```python
from build123d import *

# Parameters (mm, degrees)
SKETCH_2_R   = 5
SKETCH_2_R_2 = 2.092708753


with BuildPart() as part:
    # 扫描1: sweep along a path in 草图1
    with BuildLine(Plane.XY) as sweep_1_path:
        Line((0, 0), (0, 12))
        ThreePointArc((0, 12), (2.343145751, 17.656854249), (8, 20))
        Line((8, 20), (20, 20))
    # 草图2 → 扫描1 (sweep)
    with BuildSketch(Plane(origin=(0, 0, 0), x_dir=(1, 0, 0), z_dir=(0, 1, 0))):
        Circle(SKETCH_2_R)
        Circle(SKETCH_2_R_2, mode=Mode.SUBTRACT)
    sweep(path=sweep_1_path.line)


solid = part.part
```
Geometry: final body of the model. Coordinates: model frame, mm. A direction names the side the tool comes from. Coordinates: 2 decimals unless noted, no trailing zeros. Order: outer loops, then holes, each group sorted by start corner. A loop starts at its lowest first (then second) coordinate and runs counter-clockwise, first axis right, second up. Notation, with made-up numbers: (-34, -34.5) -> (6, -34.5) arc R20 ccw to (6, -27.5) -> close; hole circle Ø1 at (86.5, 54.5). An arc over 180 degrees is marked (long way). Answer in a Markdown table with one row per item.
Item 1: Section C-C on z = 3.5. Output: boundary loops of the cut face in (x, y).
Return value:
| item | result |
|---|---|
| outline | (-3.57, 0) -> (3.57, 0) -> (3.57, 12) arc R4.43 cw to (8, 16.43) -> (20, 16.43) -> (20, 23.57) -> (8, 23.57) arc R11.57 ccw to (-3.57, 12) -> close |
Item 2: Access query for faces 1 (the cylindrical face through (14, 25, 0)), 2 (the cylindrical face through (-0.454, 6.084, 2.043)). Directions: +Z, -Z, +X, -X, +Y, -Y. A direction counts if a zero-diameter tool reaches every point of the face in a straight line with its end or side. Return the directions, or none.
Return value:
| item | result |
|---|---|
| face 1 | +X |
| face 2 | -Y |
Item 3: Contact query for flat-ended pins moving along their axis: P1, Ø6, axis at y = 21.5, z = 0.5, coming from the -X side; P2, Ø4, axis at x = 0, z = 0, coming from the +Y side; P3, Ø1, axis at y = 19.5, z = 0, coming from the +X side; P4, Ø6, axis at y = 2.5, z = 2.5, coming from the -X side. Output: stop coordinate, or through.
Return value:
| item | result |
|---|---|
| P1 | stops at x = -3.25 |
| P2 | stops at y = 23.53 |
| P3 | stops at x = 1.85 |
| P4 | stops at x = -5 |
Item 4: Draft query along Y for faces 3 (the flat face through (-2.2, 0, 1)), 4 (the flat face through (20, 22.2, 1)), 5 (the cylindrical face through (14.08, 22.09, -0.09)). Return one class per face: released by +Y, released by -Y, zero draft, split by the parting line, or undercut.
Return value:
| item | result |
|---|---|
| face 3 | released by -Y |
| face 4 | zero draft |
| face 5 | undercut |
Item 5: Section A-A on z = 0. Output: boundary loops of the cut face in (x, y).
Return value:
| item | result |
|---|---|
| outline | (-5, 0) -> (-2.09, 0) -> (-2.09, 12) arc R10.09 cw to (8, 22.09) -> (20, 22.09) -> (20, 25) -> (8, 25) arc R13 ccw to (-5, 12) -> close; (2.09, 0) -> (5, 0) -> (5, 12) arc R3 cw to (8, 15) -> (20, 15) -> (20, 17.91) -> (8, 17.91) arc R5.91 ccw to (2.09, 12) -> close |
Item 6: Ray query, L1, parallel to X at y = 3, z = 0; L2, parallel to Y at x = 11, z = 0. Return the intervals inside material, ascending.
Return value:
| item | result |
|---|---|
| L1 | x = -5 to -2.09, 2.09 to 5 |
| L2 | y = 15 to 17.91, 22.09 to 25 |
Item 7: Section B-B on x = 8.5. Output: boundary loops of the cut face in (y, z).
Return value:
| item | result |
|---|---|
| outline | circle Ø10 at (20, 0); hole circle Ø4.19 at (20, 0) |
